from build123d import *

# Parameters (mm, degrees)
SKETCH2_W           = 44.45
SKETCH2_H           = 44.45
BOSS_EXTRUDE1_DEPTH = 50.8
SKETCH3_R           = 6.849999
CUT_EXTRUDE1_DEPTH  = 50.8
SKETCH4_R           = 3.674999
CUT_EXTRUDE2_DEPTH  = 6.35


with BuildPart() as part:
    # Sketch2 → Boss-Extrude1 (new body)
    with BuildSketch(Plane(origin=(0, 0, 0), x_dir=(1, 0, 0), z_dir=(0, 1, 0))):
        with Locations((22.225, -22.225)):
            Rectangle(SKETCH2_W, SKETCH2_H)
    extrude(amount=BOSS_EXTRUDE1_DEPTH)

    # Sketch3 → Cut-Extrude1 (cut)
    with BuildSketch(Plane.XY.offset(44.45)):
        with Locations((22.225, 25.4)):
            Circle(SKETCH3_R)
    extrude(amount=-CUT_EXTRUDE1_DEPTH, mode=Mode.SUBTRACT)

    # Sketch4 → Cut-Extrude2 (cut)
    with BuildSketch(Plane.XZ):
        with Locations(Location((11.08184529, 22.225, 0), (0, 0, 270))):  # turned: the seam where the file's is
            Circle(SKETCH4_R)
        with Locations(Location((33.401, 22.225, 0), (0, 0, 270))):  # turned: the seam where the file's is
            Circle(SKETCH4_R)
    extrude(amount=-CUT_EXTRUDE2_DEPTH, mode=Mode.SUBTRACT)


solid = part.part
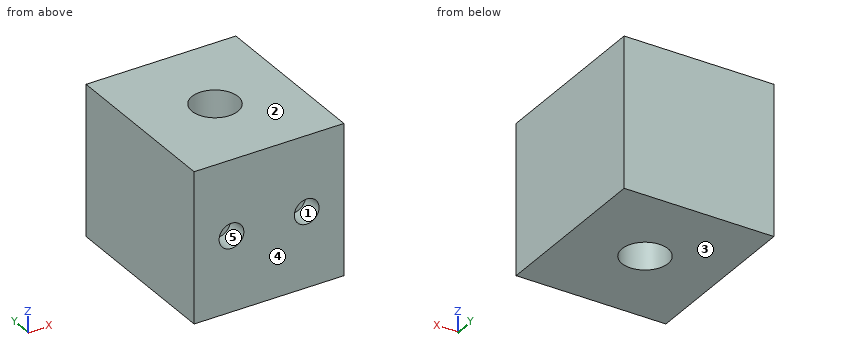
CAD build for the part. Positions are in the model's coordinates, mm. Face numbers are marked on the shaded views. A direction names the side the tool comes from. Round coordinates to 2 decimals unless told otherwise and drop trailing zeros. Write each loop counter-clockwise with the first axis right and the second up, starting at its lowest first coordinate (ties: lowest second). Pieces come first, ordered by that corner, then holes.
(1) Slice it at B-B, the plane z = 14.5. Write the cut outline in (x, y) (3 decimals), and give its area (3 significant figures).
(2) Probe line 1 along X through (y, z) = (25.5, 20.5); line 2 along X through (y, z) = (19.5, 9); line 3 along Y through (x, z) = (20, 20.5). List the from-to ranges inside material, lowest first.
(3) Drop flat-ended pins along their axis: P1, Ø11, axis at x = 22.225, y = 25.4, coming from the +Z side; P2, Ø2, axis at x = 31.5, z = 20.5, coming from the -Y side. Give the stop position or say it passes through.
(4) Slice it at C-C, the plane x = 28. Write the cut outline in (y, z).
(5) Slice it at A-A, the plane y = 25.4. Write the cut outline in (x, z) (3 decimals), and give its area (3 significant figures).
(6) Mould opens along Z. For the marked faces 1, 2 and 3 say: pulls with the +Z half, pulls with the -Z half, needs draft (parallel to the pull), parting line crosses it, or undercut.
(7) Slice it at D-D, the plane z = 23.5. Write the cut outline in (x, y) (3 decimals), and give its area (3 significant figures).
(8) 3-axis set-ups, long thin cutter, end or side, ignore diameter. For the marked faces 4 and 5: which of +Z, -Z, +X, -X, +Y, -Y reach the whole face in a straight line?
From the geometry:
1. outline: (0, 0) - (44.45, 0) - (44.45, 50.8) - (0, 50.8) - close; hole circle Ø13.7 at (22.225, 25.4)
1. area: 2,110 mm2
2. line 1: x = 0 to 15.38, 29.07 to 44.45
2. line 2: x = 0 to 18.74, 25.71 to 44.45
2. line 3: y = 0 to 18.92, 31.88 to 50.8
3. P1: passes through
3. P2: stops at y = 6.35
4. outline: (0, 0) - (21.72, 0) - (21.72, 44.45) - (0, 44.45) - close; (29.08, 0) - (50.8, 0) - (50.8, 44.45) - (29.08, 44.45) - close
5. outline: (0, 0) - (15.375, 0) - (15.375, 44.45) - (0, 44.45) - close; (29.075, 0) - (44.45, 0) - (44.45, 44.45) - (29.075, 44.45) - close
5. area: 1,370 mm2
6. face 1: undercut
6. face 2: pulls with the +Z half
6. face 3: pulls with the -Z half
7. outline: (0, 0) - (7.635, 0) - (7.635, 6.35) - (14.529, 6.35) - (14.529, 0) - (29.954, 0) - (29.954, 6.35) - (36.848, 6.35) - (36.848, 0) - (44.45, 0) - (44.45, 50.8) - (0, 50.8) - close; hole circle Ø13.7 at (22.225, 25.4)
7. area: 2,020 mm2
8. face 4: +Z, -Z, +X, -X, -Y
8. face 5: -Y
